Autodesk Inventor part; units mm, degrees
ref_plane "YZ Plane" through (0, 0, 0) normal (1, 0, 0) x (0, 1, 0)
ref_plane "XZ Plane" through (0, 0, 0) normal (0, 1, 0) x (-1, 0, 0)
ref_plane "XY Plane" through (0, 0, 0) normal (0, 0, 1) x (1, 0, 0)
sketch "Sketch1" plane through (0, 0, 0) normal (0, 1, 0) x (-1, 0, 0)
  line L0 (-38.1, 57.15) -> (38.1, 57.15)
  line L1 (38.1, 57.15) -> (38.1, -57.15)
  line L2 (38.1, -57.15) -> (-38.1, -57.15)
  line L3 (-38.1, -57.15) -> (-38.1, 57.15)
  line L4 (-38.1, 57.15) -> (38.1, -57.15) construction
  line L5 (38.1, 57.15) -> (-38.1, -57.15) construction
  line L6 (44.45, -63.5) -> (44.45, 63.5)
  line L7 (44.45, 63.5) -> (-44.45, 63.5)
  line L8 (-44.45, 63.5) -> (-44.45, -63.5)
  line L9 (-44.45, -63.5) -> (44.45, -63.5)
  point P0 (0, 0)
  dimension "d0" = 76.2
  dimension "d1" = 114.3
  dimension "d2" = 6.35
extrude "Extrusion1" add sketch "Sketch1" along normal blind 6.35
sketch "Sketch2" plane through (0, 6.35, 0) normal (0, 1, 0) x (1, 0, 0)
  line L0 (-38.1, -57.15) -> (-38.1, 57.15)
  line L1 (-38.1, 57.15) -> (38.1, 57.15)
  line L2 (38.1, 57.15) -> (38.1, -57.15)
  line L3 (38.1, -57.15) -> (-38.1, -57.15)
  line L4 (-44.45, 63.5) -> (-44.45, -63.5)
  line L5 (-44.45, -63.5) -> (44.45, -63.5)
  line L6 (44.45, -63.5) -> (44.45, 63.5)
  line L7 (44.45, 63.5) -> (-44.45, 63.5)
  point P0 (0, 0)
extrude "Extrusion2" add sketch "Sketch2" along normal mid plane 6.35 contours L0 L1 L2 L3
sketch "Sketch3" plane through (0, 9.525, 0) normal (0, 1, 0) x (1, 0, 0)
  line L0 (-38.1, 57.15) -> (-38.1, -57.15)
  line L1 (-38.1, -57.15) -> (38.1, -57.15)
  line L2 (38.1, -57.15) -> (38.1, 57.15)
  line L3 (38.1, 57.15) -> (-38.1, 57.15)
  point P0 (0, 0)
extrude "Extrusion3" add sketch "Sketch3" along normal blind 12.7
properties part number "User Control Panel - Rough"
Input: part model. Units: mm. Frame: model coordinates. A direction names the side the tool comes from. Coordinates: 2 decimals unless noted, no trailing zeros. Write each loop counter-clockwise with the first axis right and the second up, starting at its lowest first coordinate (ties: lowest second). Pieces come first, ordered by that corner, then holes. Notation, with made-up numbers: (41.5, -36.75) -> (47.5, -36.75) arc R30 cw to (47.5, -7.75) -> close; hole circle Ø8 at (-30.75, -17.75). An arc over 180 degrees is marked (long way). Answer as a JSON object with one key per item and string values.
1. Section B-B on x = 11. Return the cut outline in (y, z) (3 decimals).
Result set:
{"outline": "(0, -63.5) -> (6.35, -63.5) -> (6.35, -57.15) -> (22.225, -57.15) -> (22.225, 57.15) -> (6.35, 57.15) -> (6.35, 63.5) -> (0, 63.5) -> (0, 57.15) -> (3.175, 57.15) -> (3.175, -57.15) -> (0, -57.15) -> close"}
2. Section A-A on z = 9. Return the cut outline in (x, y) (3 decimals), then the cut area to 3 significant figures.
Result set:
{"outline": "(-44.45, 0) -> (-38.1, 0) -> (-38.1, 3.175) -> (38.1, 3.175) -> (38.1, 0) -> (44.45, 0) -> (44.45, 6.35) -> (38.1, 6.35) -> (38.1, 22.225) -> (-38.1, 22.225) -> (-38.1, 6.35) -> (-44.45, 6.35) -> close", "area": "1,530 mm2"}
3. First-contact query: P1, Ø1.5, axis at y = 17, z = -22.5, coming from the -X side; P2, Ø8, axis at y = 15.5, z = -15.5, coming from the +X side; P3, Ø12, axis at x = -5.5, z = 1.5, coming from the -Y side (3 decimals). Flat tips, straight axial feed; report the tip coordinate or a pass-through.
Result set:
{"P1": "stops at x = -38.1", "P2": "stops at x = 38.1", "P3": "stops at y = 3.175"}
4. Mould query, pull axis X, two halves, no side actions, for faces 1 (the face through (-38.1, 14, -1)), 2 (the face through (-1, 2, -57.15)), 3 (the face through (40, 0, 5)). Classes: released by +X, released by -X, zero draft, split by the parting line, or undercut.
Result set:
{"face 1": "released by -X", "face 2": "undercut", "face 3": "zero draft"}
5. Material intervals for line 1 (Z direction, x = 16.5, y = 3); line 2 (X direction, y = 1.25, z = -43.5); line 3 (Z direction, x = 1, y = 16.5), sorted ascending. Write a range as from..to.
Result set:
{"line 1": "z = -63.5..-57.15, 57.15..63.5", "line 2": "x = -44.45..-38.1, 38.1..44.45", "line 3": "z = -57.15..57.15"}
6. Access query for faces 4 (the face through (-1, 14, 57.15)), 5 (the face through (38.1, 14, 1)), 6 (the face through (1, 2, 57.15)). Directions: +Z, -Z, +X, -X, +Y, -Y. A direction counts if a zero-diameter tool reaches every point of the face in a straight line with its end or side. Return the directions, or none.
Result set:
{"face 4": "+Z, +X, -X, +Y", "face 5": "+Z, -Z, +X, +Y", "face 6": "-Y"}
7. Section C-C on y = 16.5. Return the cut outline in (x, z), then the cut area to 3 significant figures.
Result set:
{"outline": "(-38.1, -57.15) -> (38.1, -57.15) -> (38.1, 57.15) -> (-38.1, 57.15) -> close", "area": "8,710 mm2"}
